```python
from build123d import *

# Parameters (mm, degrees)
MODEL_W             = 59.689998908
MODEL_H             = 3.386668819
MODEL_H_2           = 3.3866668
BOSS_EXTRUDE1_DEPTH = 3.7
SKETCH1_W           = 5
SKETCH1_H           = 5
SKETCH1_R           = 10
SKETCH1_W_2         = 4.5
SKETCH1_H_2         = 11
CUT_EXTRUDE1_DEPTH  = 10


with BuildPart() as part:
    # Model → Boss-Extrude1 (new body)
    with BuildSketch(Plane.XY):
        Polygon((7.659321824, 131.185313162), (11.645711781, 131.185313467), (11.645711781, 123.120135193), (7.659323163, 123.120135799), (7.659323163, 114.794580784), (11.645711704, 114.794580995), (11.645711704, 106.729402721), (7.659323085, 106.729402721), (7.659322496, 101.163927511), (17.960431856, 101.163927511), (17.960431856, 105.185592023), (27.661820742, 105.185592023), (27.661820742, 101.163927511), (35.952098518, 101.163927511), (35.952098518, 105.185592023), (43.642655148, 105.185592023), (43.642655148, 101.163927511), (51.968212855, 101.163927511), (51.968212855, 105.185592023), (59.658766793, 105.185592023), (59.658766793, 101.163927511), (67.949044569, 101.163927511), (67.949044569, 105.185592023), (77.650433456, 105.185592023), (77.650433456, 101.163927511), (87.951545673, 101.163927511), (87.951545673, 106.78652537), (83.965155709, 106.78652537), (83.965155709, 115.20447842), (87.951545673, 115.204478756), (87.951545673, 123.494756532), (83.965155708, 123.494756532), (83.965155708, 131.185313162), (87.951545168, 131.185313162), (87.951545168, 139.475590938), (83.965156213, 139.475590938), (83.965156213, 147.166147568), (87.951545168, 147.166147568), (87.951545168, 155.456425344), (83.965156213, 155.456425344), (83.965156213, 163.182259213), (87.951545168, 163.182259213), (87.951545168, 171.472536989), (83.965156213, 171.472536989), (83.965156213, 179.163092274), (87.951545169, 179.163092274), (87.951545169, 187.851347209), (84.066213746, 187.851347204), (83.965155204, 195.685953684), (87.951545169, 195.685953684), (87.951544665, 201.458647414), (77.650433455, 201.458647414), (77.650433455, 205.445036033), (67.949044569, 205.445036033), (67.949044569, 201.458647414), (59.658766793, 201.458647414), (59.658766793, 205.445036033), (51.968212854, 205.445036033), (51.968212854, 201.458647414), (43.642655148, 201.458647414), (43.642655148, 205.445036033), (35.952098517, 205.445036033), (35.952098517, 201.458647414), (27.661820742, 201.458647414), (27.661820742, 205.445036033), (17.960431855, 205.445036033), (17.960431855, 201.458647414), (7.659323162, 201.458647414), (7.659321865, 195.685953684), (11.645710483, 195.685953684), (11.645711788, 187.863269672), (7.65932317, 187.863269672), (7.65932317, 179.537714657), (11.645711788, 179.537715263), (11.645711788, 171.472536989), (7.659321824, 171.472536989), (7.659321824, 163.182259214), (11.645711789, 163.182259214), (11.645711789, 155.456425344), (7.659321824, 155.456425344), (7.659321824, 147.166147568), (11.645711789, 147.166147568), (11.645711789, 139.475590938), (7.659321824, 139.475590938), align=None)
        with Locations((47.664322352, 111.627811013)):
            Rectangle(MODEL_W, MODEL_H, mode=Mode.SUBTRACT)
        with Locations((47.664322352, 191.629758602)):
            Rectangle(MODEL_W, MODEL_H_2, mode=Mode.SUBTRACT)
    extrude(amount=BOSS_EXTRUDE1_DEPTH)

    # Sketch1 → Cut-Extrude1 (cut)
    with BuildSketch(Plane.XY.offset(3.7)):
        with Locations((42.509321806, 138.321145422)):
            Rectangle(SKETCH1_W, SKETCH1_H)
        Polygon((47.509321806, 160.821145422), (47.509321806, 163.321145422), (47.509321806, 165.821145422), (42.509321806, 165.821145422), (42.509321806, 160.821145422), align=None)
        Polygon((62.509321806, 165.821145422), (62.509321806, 163.321145422), (62.509321806, 160.821145422), (67.509321806, 160.821145422), (67.509321806, 165.821145422), align=None)
        with Locations((67.509321806, 138.321145422)):
            Rectangle(SKETCH1_W, SKETCH1_H)
        with Locations((27.819322898, 163.321145422)):
            Circle(SKETCH1_R)
        with Locations((27.819322898, 138.321145422)):
            Rectangle(SKETCH1_W_2, SKETCH1_H_2)
    extrude(amount=-CUT_EXTRUDE1_DEPTH, mode=Mode.SUBTRACT)


solid = part.part
```
CAD build for the part. Positions are in the model's coordinates, mm. A direction names the side the tool comes from. Coordinates: 2 decimals unless noted, no trailing zeros. Order: outer loops, then holes, each group sorted by start corner. A loop starts at its lowest first (then second) coordinate and runs counter-clockwise, first axis right, second up. Notation, with made-up numbers: (70, 30) - (123, 30) arc R15 ccw to (123, 38) - close; hole circle Ø9 at (-2, 57). An arc over 180 degrees is marked (long way). Use a Markdown table: item, result. Add a question column.
(1) Saw through at A-A (x = 55.5). Give the cut face in (y, z), then the cut area to 3 significant figures.
(2) Which spindle directions (+Z, -Z, +X, -X, +Y, -Y) get a long thin tool onto all of the face, cutting with end or side? Do faces 1 (the face through (42, 140.821, 2)), 2 (the face through (86, 187.851, 2)), 3 (the face through (27.662, 203, 2)). Say none if no direction does.
(3) Saw through at C-C (x = 22.5). Give the cut face in (y, z), then the cut area to 3 significant figures.
(4) Drill centre lines: line 1 along X through (y, z) = (140, 1.7); line 2 along Y through (x, z) = (28, 1.35); line 3 along Y through (x, z) = (74, 0.55). Where is each one in solid material? Low to high. Write a range as [from, to].
(5) Saw through at B-B (y = 162). Give the cut face in (x, z), then the cut area to 3 significant figures.
(6) Pull direction Y, two halves, no side cores. Call faces 4 (the face through (17.819, 112, 2)), 5 (the face through (13, 101.164, 2)), 6 (the face through (32, 201.459, 2)), 7 (the face through (10, 131.185, 2)): +Y half, -Y half, draft (parallel to the pull), parting line (faces both ways), or undercut.
(7) Flat gauge pins, fed straight in: pin 1 (1 mm diameter, centred on y = 146.5, z = 2.5, fed in from -X); pin 2 (1.1 mm diameter, centred on x = 15, z = 1.5, fed in from +Y); pin 3 (1 mm diameter, centred on y = 111, z = 2, fed in from +X). Where does each tip first touch, or does it go through?
(8) Saw through at D-D (z = 2.85). Count the separate pieces of the cut face and the enclosed holes in it, then the cut area to 3 significant figures.
Solved:
| question | item | result |
|---|---|---|
| 1 | outline | (105.19, 0) - (109.93, 0) - (109.93, 3.7) - (105.19, 3.7) - close; (113.32, 0) - (189.94, 0) - (189.94, 3.7) - (113.32, 3.7) - close; (193.32, 0) - (205.45, 0) - (205.45, 3.7) - (193.32, 3.7) - close |
| 1 | area | 346 mm² |
| 2 | face 1 | +Z, -Z |
| 2 | face 2 | +Z, -Z, +X |
| 2 | face 3 | +Z, -Z, +Y |
| 3 | outline | (105.19, 0) - (109.93, 0) - (109.93, 3.7) - (105.19, 3.7) - close; (113.32, 0) - (154.85, 0) - (154.85, 3.7) - (113.32, 3.7) - close; (171.79, 0) - (189.94, 0) - (189.94, 3.7) - (171.79, 3.7) - close; (193.32, 0) - (205.45, 0) - (205.45, 3.7) - (193.32, 3.7) - close |
| 3 | area | 283 mm² |
| 4 | line 1 | x = [11.65, 25.57], [30.07, 40.01], [45.01, 65.01], [70.01, 83.97] |
| 4 | line 2 | y = [101.16, 109.93], [113.32, 132.82], [143.82, 153.32], [173.32, 189.94], [193.32, 201.46] |
| 4 | line 3 | y = [105.19, 109.93], [113.32, 189.94], [193.32, 205.45] |
| 5 | outline | (11.65, 0) - (17.91, 0) - (17.91, 3.7) - (11.65, 3.7) - close; (37.73, 0) - (42.51, 0) - (42.51, 3.7) - (37.73, 3.7) - close; (47.51, 0) - (62.51, 0) - (62.51, 3.7) - (47.51, 3.7) - close; (67.51, 0) - (83.97, 0) - (83.97, 3.7) - (67.51, 3.7) - close |
| 5 | area | 157 mm² |
| 6 | face 4 | undercut |
| 6 | face 5 | -Y half |
| 6 | face 6 | +Y half |
| 6 | face 7 | undercut |
| 7 | pin 1 | stops at x = 11.65 |
| 7 | pin 2 | stops at y = 201.46 |
| 7 | pin 3 | stops at x = 83.97 |
| 8 | separate pieces | 1 |
| 8 | enclosed holes | 8 |
| 8 | area | 6,810 mm² |
